Could you check a few things on this model? Use its own coordinates, in mm. Face numbers are marked on the shaded views. A direction names the side the tool comes from. Give positions to 0.01 mm unless a question says otherwise; leave off trailing zeros. Loops run counter-clockwise (first coordinate to the right, second up) from the corner with the lowest first, then second, coordinate; pieces in that order, holes last. Notation, with made-up numbers: (84.25, 20.5) -> (143.25, 20.5) arc R27 ccw to (143.25, 42.5) -> close; hole circle Ø1 at (-32.75, 60). An arc over 180 degrees is marked (long way). Write item = value, one per line. Start each with the question number.
1) I want a section at D-D (z = -12). List the corners of the cut face in (x, y) for me (3 decimals), and give its area (3 significant figures).
2) On a 3-axis mill with a long thin cutter (end or side, diameter ignored), from which of +Z, -Z, +X, -X, +Y, -Y can I reach the whole of each face in a straight line? I mean the marked faces 1, 2 and 3. Say none if no direction works.
3) I want a section at A-A (y = -24). List the corners of the cut face in (x, z) for me (3 decimals).
4) I want a section at C-C (x = 0). List the corners of the cut face in (y, z) for me (3 decimals), and give its area (3 significant figures).
5) I need wall thicknesses on probe 1 along Y at (x, z) = (27, 8); probe 2 along Z at (x, y) = (-17, -9); probe 3 along Y at (x, z) = (-1, -15). Which ranges of each line are inside material? Lowest first, please. Write a range as from..to.
6) I want a section at B-B (z = 5). List the corners of the cut face in (x, y) for me (3 decimals).
7) I'm going to push flat-ended pins straight in: pin 1 Ø6.5 at (y, z) = (16, 3) entering from +X; pin 2 Ø7.5 at (y, z) = (15, 28) entering from -X; pin 3 Ø6 at (x, y) = (28.58, 33.1) entering from +Z; pin 4 Ø2.5 at (y, z) = (-10.5, 5) entering from -X (3 decimals). Where does each tip first touch, or does it pass through?
from build123d import *

# Parameters (mm, degrees)
F1_DEPTH = 48.26
F3_DEPTH = 8.382
F5_DEPTH = 8.382
F6_R     = 1.8288
F7_DEPTH = 32.8422
F9_DEPTH = 57.15
F10_R    = 2.286


with BuildPart() as f1:
    # F0 (on Top) → F1 (new body)
    with BuildSketch(Plane.XY):
        with BuildLine():
            Line((-38.1, 38.1), (-38.1, -38.1))
            ThreePointArc((-38.1, -38.1), (0, -50.8), (38.1, -38.1))
            Line((38.1, -38.1), (38.1, 38.1))
            ThreePointArc((38.1, 38.1), (0, 50.8), (-38.1, 38.1))
        make_face()
    extrude(amount=-F1_DEPTH)

    # F2 (on face) → F3 (join)
    with BuildSketch(Plane.XY):
        with BuildLine():
            ThreePointArc((34.925, 36.486888), (0, 47.625), (-34.925, 36.486888))
            Line((-34.925, 36.486888), (-34.925, -36.486888))
            ThreePointArc((-34.925, -36.486888), (0, -47.625), (34.925, -36.486888))
            Line((34.925, -36.486888), (34.925, 36.486888))
        make_face()
    extrude(amount=F3_DEPTH)

    # F4 (on face) → F5 (cut, through all)
    with BuildSketch(Plane.XY.offset(8.382)):
        with BuildLine():
            ThreePointArc((-26.67, -36.395757), (-25.275443, -31.1912), (-30.48, -29.796643))
            Line((-30.48, -29.796643), (-52.477045, -42.496643))
            ThreePointArc((-52.477045, -42.496643), (-53.871602, -47.7012), (-48.667045, -49.095757))
            Line((-48.667045, -49.095757), (-26.67, -36.395757))
        make_face()
        with BuildLine():
            Line((52.477045, -42.496643), (30.48, -29.796643))
            ThreePointArc((30.48, -29.796643), (25.275443, -31.1912), (26.67, -36.395757))
            Line((26.67, -36.395757), (48.667045, -49.095757))
            ThreePointArc((48.667045, -49.095757), (53.871602, -47.7012), (52.477045, -42.496643))
        make_face()
        with BuildLine():
            Line((-52.477045, 42.496643), (-30.48, 29.796643))
            ThreePointArc((-30.48, 29.796643), (-25.275443, 31.1912), (-26.67, 36.395757))
            Line((-26.67, 36.395757), (-48.667045, 49.095757))
            ThreePointArc((-48.667045, 49.095757), (-53.871602, 47.7012), (-52.477045, 42.496643))
        make_face()
        with BuildLine():
            ThreePointArc((26.67, 36.395757), (25.275443, 31.1912), (30.48, 29.796643))
            Line((30.48, 29.796643), (52.477045, 42.496643))
            ThreePointArc((52.477045, 42.496643), (53.871602, 47.7012), (48.667045, 49.095757))
            Line((48.667045, 49.095757), (26.67, 36.395757))
        make_face()
    extrude(amount=-F5_DEPTH, mode=Mode.SUBTRACT)

    # F6 (on face) → F7 (cut)
    with BuildSketch(Plane.XY):
        with Locations((28.575, -33.0962)):
            Circle(F6_R)
        with Locations((-28.575, -33.0962)):
            Circle(F6_R)
        with Locations((28.575, 33.0962)):
            Circle(F6_R)
        with Locations((-28.575, 33.0962)):
            Circle(F6_R)
    extrude(amount=-F7_DEPTH, mode=Mode.SUBTRACT)

    # F8 (on Top) → F9 (join)
    with BuildSketch(Plane.XY):
        with BuildLine():
            ThreePointArc((-12.7, 6.35), (0, -6.35), (12.7, 6.35))
            Line((12.7, 6.35), (12.7, 31.75))
            ThreePointArc((12.7, 31.75), (0, 44.45), (-12.7, 31.75))
            Line((-12.7, 31.75), (-12.7, 6.35))
        make_face()
    extrude(amount=F9_DEPTH)

    # F10
    f10_edges = [f1.edges().sort_by_distance(p)[0] for p in [
        (12.7, 19.05, 57.15),
    ]]
    fillet(f10_edges, radius=F10_R)


solid = f1.part
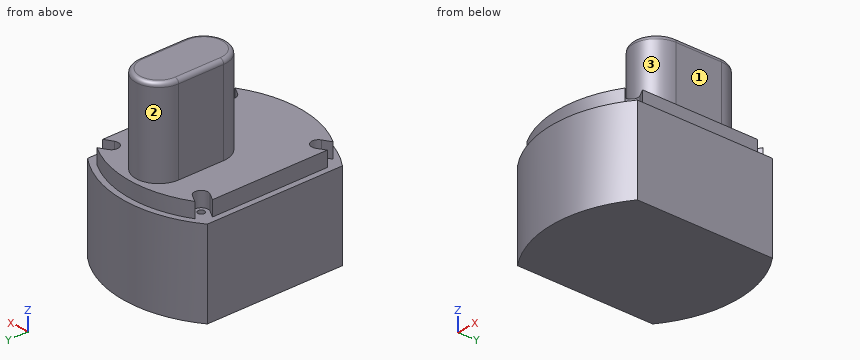
Answer list:
q1.outline = (-38.1, -38.1) arc R63.5 ccw to (38.1, -38.1) -> (38.1, 38.1) arc R63.5 ccw to (-38.1, 38.1) -> close; hole circle Ø3.658 at (-28.575, -33.096); hole circle Ø3.658 at (-28.575, 33.096); hole circle Ø3.658 at (28.575, -33.096); hole circle Ø3.658 at (28.575, 33.096)
q1.area = 7,080 mm^2
q2.face_1 = +Z, +X, +Y, -Y
q2.face_2 = +Z, +Y
q2.face_3 = +Z, -Y
q3.outline = (-38.1, -48.26) -> (38.1, -48.26) -> (38.1, 0) -> (34.925, 0) -> (34.925, 8.382) -> (-34.925, 8.382) -> (-34.925, 0) -> (-38.1, 0) -> close
q4.outline = (-50.8, -48.26) -> (50.8, -48.26) -> (50.8, 0) -> (47.625, 0) -> (47.625, 8.382) -> (44.45, 8.382) -> (44.45, 54.864) arc R2.286 ccw to (42.164, 57.15) -> (-4.064, 57.15) arc R2.286 ccw to (-6.35, 54.864) -> (-6.35, 8.382) -> (-47.625, 8.382) -> (-47.625, 0) -> (-50.8, 0) -> close
q4.area = 8,180 mm^2
q5.probe_1 = -41.25..-36.59, -29.63..29.63, 36.59..41.25
q5.probe_2 = -48.26..8.38
q5.probe_3 = -50.79..50.79
q6.outline = (-34.925, -32.363) -> (-30.48, -29.797) arc R3.81 cw to (-26.67, -36.396) -> (-31.131, -38.972) arc R60.325 ccw to (31.131, -38.972) -> (26.67, -36.396) arc R3.81 cw to (30.48, -29.797) -> (34.925, -32.363) -> (34.925, 32.363) -> (30.48, 29.797) arc R3.81 cw to (26.67, 36.396) -> (31.131, 38.972) arc R60.325 ccw to (-31.131, 38.972) -> (-26.67, 36.396) arc R3.81 cw to (-30.48, 29.797) -> (-34.925, 32.363) -> close
q7.pin_1 = 38.1
q7.pin_2 = -12.7
q7.pin_3 = 0
q7.pin_4 = -34.925
